Can you work these out from the drawing? Everything is in mm from the part's minimum corner. A direction names the side the tool comes from. Round coordinates to 2 decimals unless told otherwise and drop trailing zeros. Write each loop counter-clockwise with the first axis right and the second up, starting at its lowest first coordinate (ties: lowest second). Pieces come first, ordered by that corner, then holes. Notation, with made-up numbers: (83.25, 77.25) - (116.25, 77.25) arc R19 ccw to (116.25, 87.25) - close; hole circle Ø11 at (62.25, 41). An arc over 180 degrees is marked (long way). One line per item, written item: value. Start each with the question number.
Item 1: Imagine slicing it at D-D, the plane y = 29.5. Please give me the cut outline in (x, z), then the cut area to 3 significant figures.
Item 2: Imagine slicing it at B-B, the plane x = 10. Please give me the cut outline in (y, z).
Item 3: For P1, Ø8.5, axis at x = 14, y = 17, coming from the -Z side; P2, Ø4, axis at x = 26, y = 7.5, coming from the -Z side, each with a flat end and sliding along its axis, tell me the tip position at first contact or that it passes through.
Item 4: Imagine slicing it at A-A, the plane y = 25. Please give me the cut outline in (x, z), then the cut area to 3 significant figures.
Item 5: Imagine slicing it at C-C, the plane z = 1.2. Please give me the cut outline in (x, y), then the cut area to 3 significant figures.
Item 6: For the marked faces 1 and 2, which set-ups out of +Z, -Z, +X, -X, +Y, -Y let a thin tool reach every point of the face, with its end or its side?
Item 7: If I drill on line 1 (X direction, y = 11, z = 2.4); line 2 (Y direction, x = 26.5, z = 0.3); line 3 (X direction, y = 12.5, z = 1.6), over which ranges is the centre line in solid material (lowest first)?
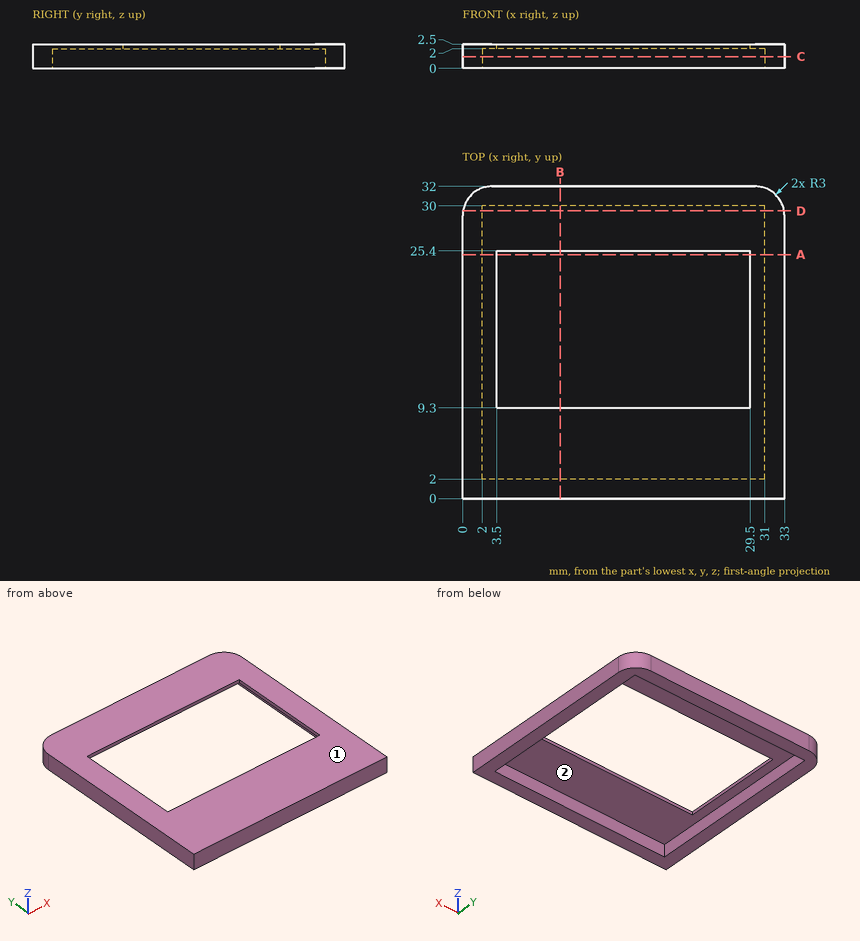
Values follow:
1. outline: (0.04, 0) - (2, 0) - (2, 2) - (31, 2) - (31, 0) - (32.96, 0) - (32.96, 2.5) - (0.04, 2.5) - close
1. area: 24.3 mm^2
2. outline: (0, 0) - (2, 0) - (2, 2) - (9.3, 2) - (9.3, 2.5) - (0, 2.5) - close; (25.4, 2) - (30, 2) - (30, 0) - (32, 0) - (32, 2.5) - (25.4, 2.5) - close
3. P1: passes through
3. P2: stops at z = 2
4. outline: (0, 0) - (2, 0) - (2, 2) - (3.5, 2) - (3.5, 2.5) - (0, 2.5) - close; (29.5, 2) - (31, 2) - (31, 0) - (33, 0) - (33, 2.5) - (29.5, 2.5) - close
4. area: 11.5 mm^2
5. outline: (0, 0) - (33, 0) - (33, 29) arc R3 ccw to (30, 32) - (3, 32) arc R3 ccw to (0, 29) - close; hole (2, 2) - (31, 2) - (31, 30) - (2, 30) - close
5. area: 240 mm^2
6. face 1: +Z, +X, -X, +Y, -Y
6. face 2: -Z
7. line 1: x = 0 to 3.5, 29.5 to 33
7. line 2: y = 0 to 2, 30 to 32
7. line 3: x = 0 to 2, 31 to 33
